Verification items for the finished model (mm, model axes). A direction names the side the tool comes from. Round coordinates to 2 decimals unless told otherwise and drop trailing zeros. Write each loop counter-clockwise with the first axis right and the second up, starting at its lowest first coordinate (ties: lowest second). Pieces come first, ordered by that corner, then holes. Notation, with made-up numbers: (16, 19) - (44, 19) arc R14 ccw to (44, 40) - close; hole circle Ø9 at (86.5, 8.25). An arc over 180 degrees is marked (long way). Answer as a JSON object with one key per item and string values. Group by question number.
1) Go/stop test with flat-tipped pins: pin 1 Ø1.5 at (x, z) = (-15.5, -4) entering from +Y; pin 2 Ø1.5 at (x, z) = (-16, -8) entering from -Y; pin 3 Ø6 at (y, z) = (-2.5, -9) entering from +X. Record where each tip stops, or that it passes through.
2) Section check D-D (x = -6). Enter the section's corners in (y, z), then the cut area to 4 significant figures.
3) Mould release check, pull along X, two halves, no side actions. Record for faces 1 (the flat face through (16, -28.25, -6)), 2 (the flat face through (14, -31.5, -5.9)), 3 (the flat face through (-17, -31.5, -5.9)): +X half, -X half, draft (parallel to the pull), parting line (faces both ways), or undercut.
4) Section check C-C (x = 0). Enter the section's corners in (y, z), then the cut area to 4 significant figures.
5) Thickness scan on line 1 (Y direction, x = 16, z = -10.25); line 2 (Y direction, x = 3, z = 0.75); line 3 (X direction, y = 4, z = -6). Record the ranges inside material, lowest first.
6) Section check A-A (z = -10). Enter the section's corners in (x, y).
7) Section check B-B (y = -30). Enter the section's corners in (x, z), then the cut area to 3 significant figures.
8) Set-up check for faces 4 (the flat face through (-7.033, 31, 1)), 5 (the flat face through (17, 32, -6)), 6 (the flat face through (16, 28.25, -6)): record each of +Z, -Z, +X, -X, +Y, -Y from which the full face is reachable in a straight line by a thin tool's end or side.
```python
from build123d import *

# Parameters (mm, degrees)
SKETCH_1_W          = 48
SKETCH_1_H          = 67
EXTRUDE_2_DEPTH     = 3
SKETCH_3_W          = 3
SKETCH_3_H          = 67
EXTRUDE_3_DEPTH     = 12
SKETCH_4_R          = 1.35
SKETCH_4_W          = 12
SKETCH_4_H          = 23
CUT_EXTRUDE_1_DEPTH = 65
SKETCH_5_W          = 18.288137738
SKETCH_5_H          = 10.5
CUT_EXTRUDE_2_DEPTH = 65
SKETCH_6_W          = 3.5
SKETCH_6_H          = 67
CUT_EXTRUDE_3_DEPTH = 65
FILLET_1_R          = 3
SKETCH_7_W          = 56
SKETCH_7_H          = 82
EXTRUDE_4_DEPTH     = 3
SKETCH_9_W          = 14.065102052
SKETCH_9_H          = 5.25
CUT_EXTRUDE_4_DEPTH = 3
SKETCH_10_R         = 1.5
CUT_EXTRUDE_5_DEPTH = 3


with BuildPart() as part:
    # 草图1 → 凸台-拉伸2 (new body)
    with BuildSketch(Plane.XY):
        Rectangle(SKETCH_1_W, SKETCH_1_H)
    extrude(amount=EXTRUDE_2_DEPTH)

    # 草图3 → 凸台-拉伸3 (add)
    with BuildSketch(Plane(origin=(0, 0, 0), x_dir=(-1, 0, 0), z_dir=(0, 0, -1))):
        with Locations((-15.5, 0)):
            Rectangle(SKETCH_3_W, SKETCH_3_H)
        with Locations((15.5, 0)):
            Rectangle(SKETCH_3_W, SKETCH_3_H)
    extrude(amount=EXTRUDE_3_DEPTH)

    # 草图4 → 切除-拉伸1 (cut)
    with BuildSketch(Plane(origin=(17, 0, 0), x_dir=(0, 0, -1), z_dir=(1, 0, 0))):
        with Locations(Location((6, 2.5, 0), (0, 0, 270))):
            Circle(SKETCH_4_R)
        with Locations(Location((6, 30, 0), (0, 0, 270))):
            Circle(SKETCH_4_R)
        with Locations(Location((6, -2.5, 0), (0, 0, 270))):
            Circle(SKETCH_4_R)
        with Locations(Location((6, -30, 0), (0, 0, 270))):
            Circle(SKETCH_4_R)
        with Locations((6, -16.75)):
            Rectangle(SKETCH_4_W, SKETCH_4_H)
        with Locations((6, 16.75)):
            Rectangle(SKETCH_4_W, SKETCH_4_H)
    extrude(amount=-CUT_EXTRUDE_1_DEPTH, mode=Mode.SUBTRACT)

    # 草图5 → 切除-拉伸2 (cut)
    with BuildSketch(Plane(origin=(0, 0, 0), x_dir=(-1, 0, 0), z_dir=(0, 0, -1))):
        Rectangle(SKETCH_5_W, SKETCH_5_H)
    extrude(amount=-CUT_EXTRUDE_2_DEPTH, mode=Mode.SUBTRACT)

    # 草图6 → 切除-拉伸3 (cut)
    with BuildSketch(Plane(origin=(0, 0, 0), x_dir=(-1, 0, 0), z_dir=(0, 0, -1))):
        with Locations((22.25, 0)):
            Rectangle(SKETCH_6_W, SKETCH_6_H)
        with Locations((-22.25, 0)):
            Rectangle(SKETCH_6_W, SKETCH_6_H)
    extrude(amount=-CUT_EXTRUDE_3_DEPTH, mode=Mode.SUBTRACT)

    # 圆角1
    fillet_1_edges = [part.edges().sort_by_distance(p)[0] for p in [
        (20.5, 33.5, 1.5),
        (20.5, -33.5, 1.5),
        (-20.5, -33.5, 1.5),
        (-20.5, 33.5, 1.5),
    ]]
    fillet(fillet_1_edges, radius=FILLET_1_R)

    # 草图7 → 凸台-拉伸4 (add)
    with BuildSketch(Plane.XY.offset(3)):
        Rectangle(SKETCH_7_W, SKETCH_7_H)
    extrude(amount=-EXTRUDE_4_DEPTH)

    # 草图9 → 切除-拉伸4 (cut)
    with BuildSketch(Plane(origin=(0, 0, 0), x_dir=(-1, 0, 0), z_dir=(0, 0, -1))):
        with Locations((0, 30.875)):
            Rectangle(SKETCH_9_W, SKETCH_9_H)
        Polygon((0, -28.25), (-7.032551026, -28.25), (-7.032551026, -33.5), (7.032551026, -33.5), (7.032551026, -28.25), align=None)
    extrude(amount=-CUT_EXTRUDE_4_DEPTH, mode=Mode.SUBTRACT)

    # 草图10 → 切除-拉伸5 (cut)
    with BuildSketch(Plane.XY.offset(3)):
        with Locations((0, 37.483485188)):
            Circle(SKETCH_10_R)
    extrude(amount=-CUT_EXTRUDE_5_DEPTH, mode=Mode.SUBTRACT)


solid = part.part
```
Returned:
{
 "1": {"pin 1": "y = 33.5", "pin 2": "y = -33.5", "pin 3": "x = 17"},
 "2": {"outline": "(-41, 0) - (-33.5, 0) - (-33.5, 3) - (-41, 3) - close; (-28.25, 0) - (28.25, 0) - (28.25, 3) - (-28.25, 3) - close; (33.5, 0) - (41, 0) - (41, 3) - (33.5, 3) - close", "area": "214.5 mm2"},
 "3": {"face 1": "draft", "face 2": "undercut", "face 3": "-X half"},
 "4": {"outline": "(-41, 0) - (-33.5, 0) - (-33.5, 3) - (-41, 3) - close; (-28.25, 0) - (28.25, 0) - (28.25, 3) - (-28.25, 3) - close; (33.5, 0) - (35.98, 0) - (35.98, 3) - (33.5, 3) - close; (38.98, 0) - (41, 0) - (41, 3) - (38.98, 3) - close", "area": "205.5 mm2"},
 "5": {"line 1": "-33.5 to -28.25, -5.25 to 5.25, 28.25 to 33.5", "line 2": "-41 to -33.5, -28.25 to 28.25, 33.5 to 41", "line 3": "-17 to -14, 14 to 17"},
 "6": {"outline": "(-17, -33.5) - (-14, -33.5) - (-14, -28.25) - (-17, -28.25) - close; (-17, -5.25) - (-14, -5.25) - (-14, 5.25) - (-17, 5.25) - close; (-17, 28.25) - (-14, 28.25) - (-14, 33.5) - (-17, 33.5) - close; (14, -33.5) - (17, -33.5) - (17, -28.25) - (14, -28.25) - close; (14, -5.25) - (17, -5.25) - (17, 5.25) - (14, 5.25) - close; (14, 28.25) - (17, 28.25) - (17, 33.5) - (14, 33.5) - close"},
 "7": {"outline": "(-28, 0) - (-17, 0) - (-17, -4.65) - (-14, -4.65) - (-14, 0) - (-7.03, 0) - (-7.03, 3) - (-28, 3) - close; (-17, -12) - (-14, -12) - (-14, -7.35) - (-17, -7.35) - close; (7.03, 0) - (14, 0) - (14, -4.65) - (17, -4.65) - (17, 0) - (28, 0) - (28, 3) - (7.03, 3) - close; (14, -12) - (17, -12) - (17, -7.35) - (14, -7.35) - close", "area": "182 mm2"},
 "8": {"face 4": "+Z, -Z", "face 5": "-Z, +X, +Y, -Y", "face 6": "-Z, +X, -X"}
}
